from build123d import *

# Parameters (mm, degrees)
SKETCH1_R           = 3
BOSS_EXTRUDE1_DEPTH = 2.5
BOSS_EXTRUDE2_START = 2.5
SKETCH1_3_R         = 4
BOSS_EXTRUDE2_DEPTH = 2.5
BOSS_EXTRUDE3_DEPTH = 16


with BuildPart() as part:
    # Sketch1 → Boss-Extrude1 (new body)
    with BuildSketch(Plane(origin=(0, 0, 0), x_dir=(1, 0, 0), z_dir=(0, 1, 0))):
        with BuildLine():
            Line((22.75, -8), (45.5, -8))
            ThreePointArc((45.5, -8), (53.5, 0), (45.5, 8))
            Line((45.5, 8), (22.75, 8))
            Line((22.75, 8), (22.75, -8))
        make_face()
        with Locations(Location((45.5, 0, 0), (0, 0, 270))):
            Circle(SKETCH1_R, mode=Mode.SUBTRACT)
    extrude(amount=BOSS_EXTRUDE1_DEPTH)



with BuildPart() as body_2:
    # Sketch1<3> → Boss-Extrude2 (new body)
    with BuildSketch(Plane(origin=(0, 0, 0), x_dir=(1, 0, 0), z_dir=(0, 1, 0)).offset(BOSS_EXTRUDE2_START)):
        with BuildLine():
            Line((0, -8), (22.75, -8))
            Line((22.75, -8), (22.75, 8))
            Line((22.75, 8), (15.305028665, 8))
            ThreePointArc((15.305028665, 8), (10.877839941, 9.950308654), (9.328779377, 14.533333333))
            Line((9.328779377, 14.533333333), (11.952427887, 43.93254122))
            Line((11.952427887, 43.93254122), (11.952498577, 43.933333333))
            ThreePointArc((11.952498577, 43.933333333), (0, 57), (-11.952498577, 43.933333333))
            Line((-11.952498577, 43.933333333), (-7.968332384, -0.711111111))
            ThreePointArc((-7.968332384, -0.711111111), (-5.399588462, -5.902918299), (0, -8))
        make_face()
        with Locations(Location((0, 0, 0), (0, 0, 270))):
            Circle(SKETCH1_3_R, mode=Mode.SUBTRACT)
        with Locations(Location((0, 45, 0), (0, 0, 270))):
            Circle(SKETCH1_3_R, mode=Mode.SUBTRACT)
    extrude(amount=BOSS_EXTRUDE2_DEPTH)


with BuildPart() as part_1:
    add(part.part)

    add(body_2.part)  # Boss-Extrude3 merges body 2
    # Sketch2 → Boss-Extrude3 (add)
    with BuildSketch(Plane.XY.offset(8)):
        with BuildLine():
            Line((22.75, 5), (19.25, 5))
            Line((19.25, 5), (19.25, 2.5))
            ThreePointArc((19.25, 2.5), (20.744035762, 2.004459314), (21.645787119, 0.714285714))
            ThreePointArc((21.645787119, 0.714285714), (22.006487662, 0.198216274), (22.604101966, 0))
            Line((22.604101966, 0), (22.75, 0))
            Line((22.75, 0), (22.75, 2.5))
            Line((22.75, 2.5), (26.104101966, 2.5))
            ThreePointArc((26.104101966, 2.5), (25.506487662, 2.698216274), (25.145787119, 3.214285714))
            ThreePointArc((25.145787119, 3.214285714), (24.244035762, 4.504459314), (22.75, 5))
        make_face()
    extrude(amount=-BOSS_EXTRUDE3_DEPTH)


with BuildPart() as body_2_2:
    # Mirror4: mirrored copy
    add(part_1.part.mirror(Plane.ZX))


solid = body_2_2.part
The listing builds one solid part. Answer for the finished solid, in the listing's coordinates (mm). A direction names the side the tool comes from. Give positions to 0.01 mm unless a question says otherwise; leave off trailing zeros. Write each loop counter-clockwise with the first axis right and the second up, starting at its lowest first coordinate (ties: lowest second). Pieces come first, ordered by that corner, then holes.
1) Section A-A (z = -45) is taken. Write down the section's boundary in (x, y).
2) Given P1, Ø2, axis at x = -4, y = -3.5, coming from the -Z side; P2, Ø8, axis at x = 33, z = -3.5, coming from the -Y side; P3, Ø6, axis at x = 13.5, z = -4, coming from the +Y side; P4, Ø10.5, axis at x = 0, z = -45, coming from the -Y side, each flat-ended and moving along its own axis, determine where each tip first touches the part or whether it passes through.
3) For a pull along X with two mould halves and no side action, classify faces 1 (the face through (48.474, -1.232, -0.391)), 2 (the face through (20.726, -2.018, 0.112)), 3 (the face through (53.498, -1.232, 0.176)) as pulls with the +X half, pulls with the -X half, needs draft (parallel to the pull), parting line crosses it, or undercut.
4) Section B-B (x = 29) is taken. Write down the section's boundary in (y, z), and give its area (3 significant figures).
5) A tool of negligible diameter and unlimited length cuts with its end or side. For faces 4 (the face through (31, -2, -8)), 5 (the face through (3, -2.5, -25)), 6 (the face through (-9.988, -3.732, -21.924)), 7 (the face through (40, -2.5, 0)), from which of +Z, -Z, +X, -X, +Y, -Y can it reach the whole face along a straight path? Write none if from no direction.
6) Find the intervals of material crossed by L1, parallel to Y at x = -2, z = -19.5; L2, parallel to X at y = -4, z = -47; L3, parallel to X at y = -3.1, z = -42.5, in increasing order.
7) Section C-C (z = -32.5) is taken. Write down the section's boundary in (x, y), and give its area (3 significant figures).
Response:
1. outline: (-12, -5) - (-4, -5) - (-4, -2.5) - (-12, -2.5) - close; (4, -5) - (12, -5) - (12, -2.5) - (4, -2.5) - close
2. P1: stops at z = -56.62
2. P2: stops at y = -2.5
2. P3: stops at y = -2.5
2. P4: stops at y = -5
3. face 1: undercut
3. face 2: pulls with the -X half
3. face 3: pulls with the +X half
4. outline: (-2.5, -8) - (0, -8) - (0, 8) - (-2.5, 8) - close
4. area: 40.0 mm2
5. face 4: -Z, +X, +Y, -Y
5. face 5: +Z, -Z, -X, +Y
5. face 6: +Z, -X, +Y, -Y
5. face 7: +Z, -Z, +X, -Y
6. L1: y = -5 to -2.5
6. L2: x = -11.83 to -3.46, 3.46 to 11.83
6. L3: x = -11.82 to -3.12, 3.12 to 11.82
7. outline: (-10.93, -5) - (10.93, -5) - (10.93, -2.5) - (-10.93, -2.5) - close
7. area: 54.7 mm2
